from build123d import *

# Parameters (mm, degrees)
SKETCH1_W           = 50
SKETCH1_H           = 10
BOSS_EXTRUDE1_DEPTH = 50
SKETCH2_R           = 5
BOSS_EXTRUDE2_DEPTH = 2
LPATTERN1_COUNT     = 10
LPATTERN1_PITCH     = 50


with BuildPart() as part:
    # Sketch1 → Boss-Extrude1 (new body)
    with BuildSketch(Plane.XY):
        Rectangle(SKETCH1_W, SKETCH1_H)
    boss_extrude1 = extrude(amount=BOSS_EXTRUDE1_DEPTH)

    # Sketch2 → Boss-Extrude2 (add)
    with BuildSketch(Plane.XZ.offset(5)):
        with BuildLine():
            Line((-50, 10), (-25, 10))
            Line((-25, 10), (-25, 40))
            Line((-25, 40), (-50, 40))
            add(Edge.make_bspline(
                [(-50, 40), (-64.127186128, 28.759951739), (-81.969053702, 25)],
                knots=[0, 0, 0, 1, 1, 1], degree=2))
            add(Edge.make_bspline(
                [(-50, 10), (-64.127186128, 21.240048261), (-81.969053702, 25)],
                knots=[0, 0, 0, 1, 1, 1], degree=2))
        make_face()
        with Locations((-50, 25)):
            Circle(SKETCH2_R, mode=Mode.SUBTRACT)
    boss_extrude2 = extrude(amount=-BOSS_EXTRUDE2_DEPTH)

    # LPattern1: Boss-Extrude1, Boss-Extrude2 ×10
    with Locations(*[(0, 0, i * LPATTERN1_PITCH) for i in range(1, LPATTERN1_COUNT)]):
        add(boss_extrude1)
        add(boss_extrude2)


solid = part.part
Design review of the part built by this model. Coordinates are the model's own, in mm. A direction names the side the tool comes from. Coordinates: 2 decimals unless noted, no trailing zeros. Loops run counter-clockwise (first coordinate to the right, second up) from the corner with the lowest first, then second, coordinate; pieces in that order, holes last. Notation, with made-up numbers: M 30.5,52 L 65.5,52 A11 cw 65.5,61 Z; hole C 25,-36 d7. An arc over 180 degrees is marked long. Answer as CSV lines item,"result".
Item 1: Add section B-B on z = 303.5. State the section outline as (x, y) points, plus the area to 3 significant figures.
Answer list:
outline,"M -25,-5 L 25,-5 L 25,5 L -25,5 Z"
area,"500 mm²"
Item 2: For probe 1 along X at (y, z) = (-1, 408); probe 2 along X at (y, z) = (-3.5, 269), list the stretches that pass through material, from the lowest coordinate up.
Answer list:
probe 1,"-25 to 25"
probe 2,"-64.28 to 25"
Item 3: The part is to be moulded in two halves that separate along Z. For faces 1 (the face through (-50.651, -4.014, 429.957)), 2 (the face through (0, 0, 0)), 3 (the face through (-50.651, -4.014, 379.957)), 4 (the face through (-41, -3, 275)), say which applies: pulls with the +Z half, pulls with the -Z half, needs draft (parallel to the pull), parting line crosses it, or undercut.
Answer list:
face 1,"undercut"
face 2,"pulls with the -Z half"
face 3,"undercut"
face 4,"needs draft"
Item 4: Machinability: for faces 5 (the face through (-41, -3, 325)), 6 (the face through (0, 0, 500)), which of the approach directions +Z, -Z, +X, -X, +Y, -Y give a long, thin tool a straight path to every point of the face, cutting with its end or side? Answer none if there is none.
Answer list:
face 5,"+Z, -Z, -X, +Y"
face 6,"+Z, +X, -X, +Y, -Y"
Item 5: Add section A-A on x = -32.5. Count the separate pieces of the cut face and the enclosed holes in it, plus the area to 3 significant figures.
Answer list:
separate pieces,"10"
enclosed holes,"0"
area,"600 mm²"
Item 6: Add section C-C on y = -0.5. State the section outline as (x, z) points.
Answer list:
outline,"M -25,0 L 25,0 L 25,500 L -25,500 Z"
Item 7: For P1, Ø24, axis at x = -41.5, z = 68.5, coming from the +Y side; P2, Ø0.6, axis at x = -36.5, y = -3.5, coming from the +Z side; P3, Ø9, axis at x = -50, z = 175, coming from the +Y side; P4, Ø0.6, axis at x = -34.5, y = -4.5, coming from the -Z side, all flat-tipped, find the tip position at first contact; note any pin that passes through.
Answer list:
P1,"y = -3"
P2,"z = 490"
P3,"through"
P4,"z = 10"
